Answer from the drawing. Dimensions are ordinates in mm from the lowest x, y and z of the part. Give positions to 0.01 mm unless a question says otherwise; leave off trailing zeros. Loops run counter-clockwise (first coordinate to the right, second up) from the corner with the lowest first, then second, coordinate; pieces in that order, holes last. Notation, with made-up numbers: (1.25, 57) - (39.25, 57) arc R27 ccw to (39.25, 80) - close; hole circle Ø8 at (12.5, 88.5). An arc over 180 degrees is marked (long way). Answer as CSV lines item,"result". Start each with the question number.
1) A cutting plane is placed at A-A (z = 18). Determine the outline of the cut face in (x, y).
2) Flat-ended cylindrical pins translate along their axes: pin 1 (4 mm diameter, centred on x = 10.5, z = 22.5, fed in from -Y); pin 2 (5 mm diameter, centred on x = 14, z = 18, fed in from +Y). Find the tip coordinate at first contact, or state that the pin passes through.
3) A cutting plane is placed at B-B (x = 14). Determine the outline of the cut face in (y, z).
4) A cutting plane is placed at C-C (y = 0.9). Determine the outline of the cut face in (x, z), and give its area (3 significant figures).
5) Find the intervals of material crossed by line 1 along X through (y, z) = (1.2, 18); line 2 along Z through (x, y) = (14, 0.8); line 3 along X through (y, z) = (0.8, 3), in increasing order.
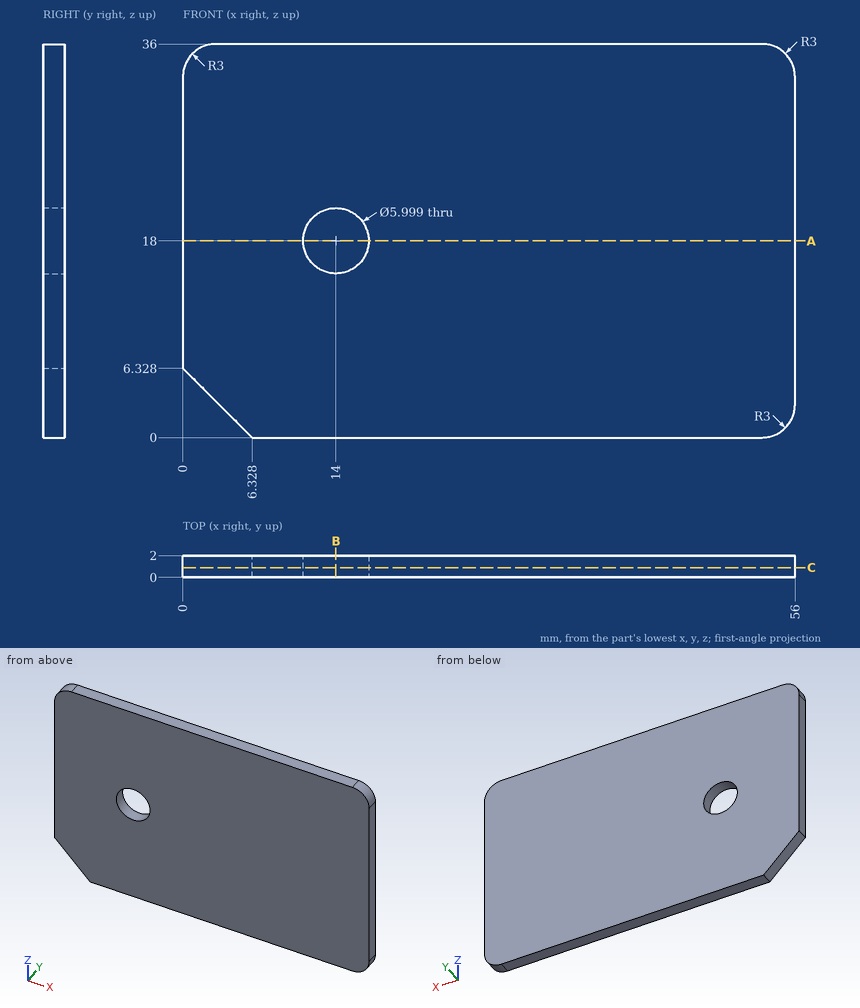
Ans:
1,outline,"(0, 0) - (11, 0) - (11, 2) - (0, 2) - close; (17, 0) - (56, 0) - (56, 2) - (17, 2) - close"
2,pin 1,"y = 0"
2,pin 2,"through"
3,outline,"(0, 0) - (2, 0) - (2, 15) - (0, 15) - close; (0, 21) - (2, 21) - (2, 36) - (0, 36) - close"
4,outline,"(0, 6.33) - (6.33, 0) - (53, 0) arc R3 ccw to (56, 3) - (56, 33) arc R3 ccw to (53, 36) - (3, 36) arc R3 ccw to (0, 33) - close; hole circle Ø6 at (14, 18)"
4,area,"1,960 mm2"
5,line 1,"0 to 11, 17 to 56"
5,line 2,"0 to 15, 21 to 36"
5,line 3,"3.33 to 56"
